Verification items for the finished model (mm, model axes). Face numbers are marked on the shaded views. A direction names the side the tool comes from. Round coordinates to 2 decimals unless told otherwise and drop trailing zeros. Write each loop counter-clockwise with the first axis right and the second up, starting at its lowest first coordinate (ties: lowest second). Pieces come first, ordered by that corner, then holes. Notation, with made-up numbers: (-31, 85) -> (18, 85) arc R21 cw to (18, 112) -> close; hole circle Ø6 at (-5.75, 40.25). An arc over 180 degrees is marked (long way). Answer as a JSON object with one key per item and string values. Group by question number.
(1) Sectioned sample at C-C on z = 1.5. Record the cut outline in (x, y).
(2) Scan lines: L1, parallel to Y at x = 0, z = 6; L2, parallel to Y at x = -5, z = 1.35; L3, parallel to X at y = -11, z = 2.75. Record each from-to range of solid material in increasing order. Write a range as from..to.
(3) Set-up check for the marked faces 1 and 2: record each of +Z, -Z, +X, -X, +Y, -Y from which the full face is reachable in a straight line by a thin tool's end or side.
(4) Sectioned sample at D-D on y = 0. Record the cut outline in (x, z), and give its area (3 significant figures).
(5) Gauge pin test, flat ends, axial feed: pin 1 Ø6 at (x, z) = (4, 10.5) entering from +Y; pin 2 Ø1.5 at (x, y) = (-5, 10) entering from +Z; pin 3 Ø10 at (x, z) = (5, 9.5) entering from +Y; pin 4 Ø3 at (x, y) = (5, 10) entering from +Z. Record the tip position at first contact, or that the pin passes through.
(6) Draft check along X on the marked faces 3, 4 and 5. Enter one of: released by +X, released by -X, zero draft, split by the parting line, or undercut.
(7) Sectioned sample at B-B on y = -10. Record the cut outline in (x, z).
(8) Sectioned sample at A-A on x = 0. Record the cut outline in (y, z), and give its area (3 significant figures).
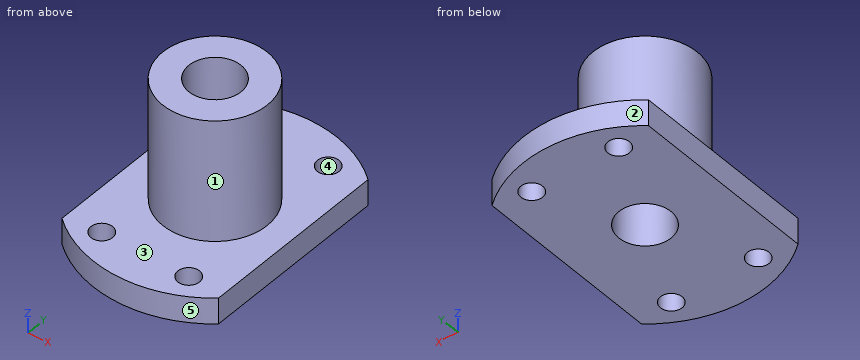
```python
from build123d import *

# Parameters (mm, degrees)
SKETCH1_R               = 3
SKETCH1_R_2             = 1.25
BOSS_EXTRUDE1_DEPTH     = 3
SKETCH2_R               = 6
SKETCH2_R_2             = 3
LINEARBALLSUPPORT_DEPTH = 14


with BuildPart() as part:
    # Sketch1 → Boss-Extrude1 (new body)
    with BuildSketch(Plane.XY):
        with BuildLine():
            Line((-9, 10.723805295), (-9, -10.723805295))
            ThreePointArc((-9, -10.723805295), (0, -14), (9, -10.723805295))
            Line((9, -10.723805295), (9, 10.723805295))
            ThreePointArc((9, 10.723805295), (0, 14), (-9, 10.723805295))
        make_face()
        Circle(SKETCH1_R, mode=Mode.SUBTRACT)
        with Locations((-5, 10)):
            Circle(SKETCH1_R_2, mode=Mode.SUBTRACT)
        with Locations((5, 10)):
            Circle(SKETCH1_R_2, mode=Mode.SUBTRACT)
        with Locations((-5, -10)):
            Circle(SKETCH1_R_2, mode=Mode.SUBTRACT)
        with Locations((5, -10)):
            Circle(SKETCH1_R_2, mode=Mode.SUBTRACT)
    extrude(amount=BOSS_EXTRUDE1_DEPTH)

    # Sketch2 → LinearBallSupport (add)
    with BuildSketch(Plane.XY.offset(3)):
        Circle(SKETCH2_R)
        Circle(SKETCH2_R_2, mode=Mode.SUBTRACT)
    extrude(amount=LINEARBALLSUPPORT_DEPTH)


solid = part.part
```
Computed values:
{
 "1": {"outline": "(-9, -10.72) arc R14 ccw to (9, -10.72) -> (9, 10.72) arc R14 ccw to (-9, 10.72) -> close; hole circle Ø2.5 at (-5, -10); hole circle Ø2.5 at (-5, 10); hole circle Ø6 at (0, 0); hole circle Ø2.5 at (5, -10); hole circle Ø2.5 at (5, 10)"},
 "2": {"L1": "-6..-3, 3..6", "L2": "-13.08..-11.25, -8.75..8.75, 11.25..13.08", "L3": "-8.66..-5.75, -4.25..4.25, 5.75..8.66"},
 "3": {"face 1": "+Z", "face 2": "+Z, -Z, +Y"},
 "4": {"outline": "(-9, 0) -> (-3, 0) -> (-3, 17) -> (-6, 17) -> (-6, 3) -> (-9, 3) -> close; (3, 0) -> (9, 0) -> (9, 3) -> (6, 3) -> (6, 17) -> (3, 17) -> close", "area": "120 mm2"},
 "5": {"pin 1": "y = 5.92", "pin 2": "through", "pin 3": "y = 6", "pin 4": "z = 3"},
 "6": {"face 3": "zero draft", "face 4": "undercut", "face 5": "split by the parting line"},
 "7": {"outline": "(-9, 0) -> (-6.25, 0) -> (-6.25, 3) -> (-9, 3) -> close; (-3.75, 0) -> (3.75, 0) -> (3.75, 3) -> (-3.75, 3) -> close; (6.25, 0) -> (9, 0) -> (9, 3) -> (6.25, 3) -> close"},
 "8": {"outline": "(-14, 0) -> (-3, 0) -> (-3, 17) -> (-6, 17) -> (-6, 3) -> (-14, 3) -> close; (3, 0) -> (14, 0) -> (14, 3) -> (6, 3) -> (6, 17) -> (3, 17) -> close", "area": "150 mm2"}
}
